Check sheet for the drawn part. Datum: minimum x, y, z corner. Units: mm. A direction names the side the tool comes from. Coordinates: 2 decimals unless noted, no trailing zeros. Loops run counter-clockwise (first coordinate to the right, second up) from the corner with the lowest first, then second, coordinate; pieces in that order, holes last.
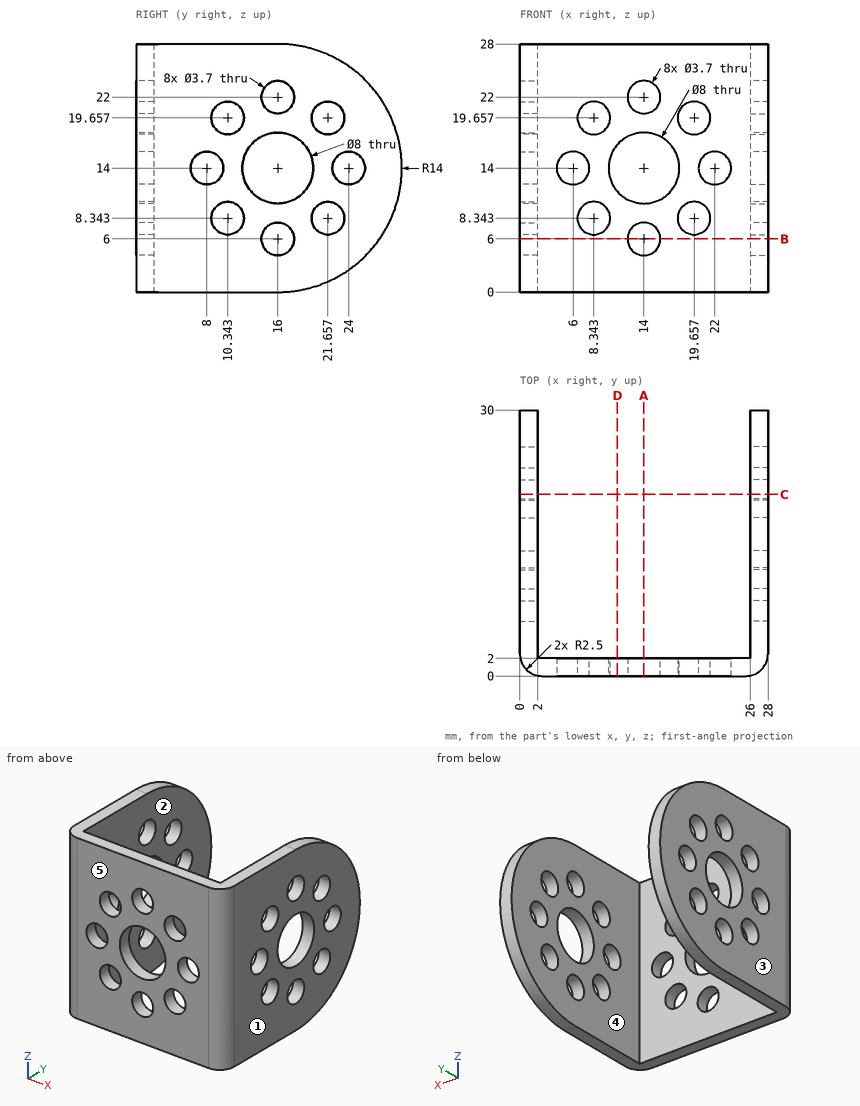
(1) Sectioned sample at D-D on x = 11. Record the cut outline in (y, z).
Findings:
outline: (0, 0) - (2, 0) - (2, 11.35) - (0, 11.35) - close; (0, 16.65) - (2, 16.65) - (2, 28) - (0, 28) - close
(2) Gauge pin test, flat ends, axial feed: pin 1 Ø3.5 at (y, z) = (10.34, 19.66) entering from -X; pin 2 Ø12 at (x, z) = (15.5, 8.5) entering from +Y; pin 3 Ø8 at (x, z) = (4.5, 9.5) entering from +Y. Record the tip position at first contact, or that the pin passes through.
Findings:
pin 1: passes through
pin 2: stops at y = 2
pin 3: stops at y = 29.93
(3) Access from +Z, -Z, +X, -X, +Y, -Y to the whole of each face (thin tool, end or side, straight path). Record for the marked faces 4 and 5.
Findings:
face 4: +Z, -Z, +Y
face 5: +Z, -Z, +X, -X, -Y
(4) Sectioned sample at B-B on z = 6. Record the cut outline in (x, y).
Findings:
outline: (0, 2.5) arc R2.5 ccw to (2.5, 0) - (12.15, 0) - (12.15, 2) - (2, 2) - (2, 14.15) - (0, 14.15) - close; (0, 17.85) - (2, 17.85) - (2, 27.49) - (0, 27.49) - close; (15.85, 0) - (25.5, 0) arc R2.5 ccw to (28, 2.5) - (28, 14.15) - (26, 14.15) - (26, 2) - (15.85, 2) - close; (26, 17.85) - (28, 17.85) - (28, 27.49) - (26, 27.49) - close
(5) Scan lines: L1, parallel to X at y = 12, z = 17.75; L2, parallel to Y at x = 27.15, z = 14; L3, parallel to Y at x = 1.6, z = 14. Record each from-to range of solid material in increasing order.
Findings:
L1: x = 0 to 2, 26 to 28
L2: y = 0.62 to 6.15, 9.85 to 12, 20 to 22.15, 25.85 to 30
L3: y = 0.17 to 6.15, 9.85 to 12, 20 to 22.15, 25.85 to 30
(6) Sectioned sample at A-A on x = 14. Record the cut outline in (y, z), and give its area (3 significant figures).
Findings:
outline: (0, 0) - (2, 0) - (2, 4.15) - (0, 4.15) - close; (0, 7.85) - (2, 7.85) - (2, 10) - (0, 10) - close; (0, 18) - (2, 18) - (2, 20.15) - (0, 20.15) - close; (0, 23.85) - (2, 23.85) - (2, 28) - (0, 28) - close
area: 25.2 mm2
(7) Draft check along X on the marked faces 1, 2 and 3. Enter one of: +X half, -X half, draft (parallel to the pull), parting line (faces both ways), or undercut.
Findings:
face 1: +X half
face 2: undercut
face 3: -X half
(8) Sectioned sample at C-C on y = 20.5. Record the cut outline in (x, z).
Findings:
outline: (0, 0.74) - (2, 0.74) - (2, 6.9) - (0, 6.9) - close; (0, 9.79) - (2, 9.79) - (2, 18.21) - (0, 18.21) - close; (0, 21.1) - (2, 21.1) - (2, 27.26) - (0, 27.26) - close; (26, 0.74) - (28, 0.74) - (28, 6.9) - (26, 6.9) - close; (26, 9.79) - (28, 9.79) - (28, 18.21) - (26, 18.21) - close; (26, 21.1) - (28, 21.1) - (28, 27.26) - (26, 27.26) - close
